Read the model definition and answer for the solid it produces. Units are mm, in the model's axes. A direction names the side the tool comes from. Coordinates: 2 decimals unless noted, no trailing zeros. Write each loop counter-clockwise with the first axis right and the second up, starting at its lowest first coordinate (ties: lowest second). Pieces come first, ordered by that corner, then holes.
(1) Straight lines are drawn through the part: line 1 along Z through (x, y) = (-37, -0.45); line 2 along X through (y, z) = (-1.2, 22.35); line 3 along Y through (x, z) = (66.2, 37.9). For each, find the intervals that lie inside material, in ascending order.
(2) Which of the six approach directions +Z, -Z, +X, -X, +Y, -Y give full straight-line access (tool end or side, diameter ignored) to faces 4 (the flat face through (0, 0, 20.75)), 5 (the flat face through (27, 0, 2)), 6 (the flat face through (67, 0, 24))?
(3) The part is cut by section A-A, the plane y = -0.95. Determine the outline of the cut face in (x, z).
(4) Determine the mould class of faces 1 (the flat face through (-5.1, 0, 23)), 2 (the flat face through (-47, 0, 0)), 3 (the flat face through (-27, 0, 2)) for opening direction Z: pulls with the +Z half, pulls with the -Z half, needs draft (parallel to the pull), parting line crosses it, or undercut.
(5) The part is cut by section B-B, the plane x = 8. Determine the outline of the cut face in (y, z), and give its area (3 significant figures).
(6) Given pin 1 (1.5 mm diameter, centred on x = -1.5, y = 0, fed in from -Z), flat-ended and moving along its own axis, determine where the tip first touches the part or whether it passes through.
```python
from build123d import *

# Parameters (mm, degrees)
SKETCH_1_W          = 134
SKETCH_1_H          = 3
EXTRUDE_1_DEPTH     = 47.9
SKETCH_4_R          = 0.7
SKETCH_4_W          = 10.2
SKETCH_4_H          = 4.7
SKETCH_4_W_2        = 54
SKETCH_4_H_2        = 3
CUT_EXTRUDE_1_DEPTH = 83.416078528
SKETCH_4_3_R        = 1
SKETCH_4_3_R_2      = 0.7
SKETCH_4_3_W        = 10.2
SKETCH_4_3_H        = 4.7
SKETCH_4_3_W_2      = 54
SKETCH_4_3_H_2      = 3
CUT_EXTRUDE_2_DEPTH = 1.5
SKETCH_5_R          = 0.35
CUT_EXTRUDE_3_DEPTH = 1.5
SKETCH_6_R          = 0.35
CUT_EXTRUDE_4_DEPTH = 1.5
SKETCH_7_R          = 0.35
CUT_EXTRUDE_5_DEPTH = 1.5
CUT_EXTRUDE_START   = -132.5
SKETCH_7_3_R        = 0.35
CUT_EXTRUDE_6_DEPTH = 1.5


with BuildPart() as part:
    # 草图1 → 凸台-拉伸1 (new body)
    with BuildSketch(Plane.XY):
        Rectangle(SKETCH_1_W, SKETCH_1_H)
    extrude(amount=EXTRUDE_1_DEPTH)

    # 草图4 → 切除-拉伸1 (cut, through all)
    with BuildSketch(Plane(origin=(0, 1.5, 0), x_dir=(1, 0, 0), z_dir=(0, 1, 0))):
        with Locations(Location((37, -46.4, 0), (0, 0, 270))):
            Circle(SKETCH_4_R)
        with Locations(Location((-37, -46.4, 0), (0, 0, 270))):
            Circle(SKETCH_4_R)
        with Locations((0, -23.1)):
            Rectangle(SKETCH_4_W, SKETCH_4_H)
        with Locations((0, -1.5)):
            Rectangle(SKETCH_4_W_2, SKETCH_4_H_2)
        with Locations(Location((-37, -1.5, 0), (0, 0, 270))):
            Circle(SKETCH_4_R)
        with Locations(Location((37, -1.5, 0), (0, 0, 270))):
            Circle(SKETCH_4_R)
    extrude(amount=-CUT_EXTRUDE_1_DEPTH, mode=Mode.SUBTRACT)

    # 草图4<3> → 切除-拉伸2 (cut)
    # profile 1 of 6: a face of its own
    with BuildSketch(Plane(origin=(0, 1.5, 0), x_dir=(1, 0, 0), z_dir=(0, 1, 0))):
        with Locations(Location((-37, -46.4, 0), (0, 0, 270))):
            Circle(SKETCH_4_3_R)
        with Locations(Location((-37, -46.4, 0), (0, 0, 270))):
            Circle(SKETCH_4_3_R_2, mode=Mode.SUBTRACT)
    # profile 2 of 6: a face of its own
    with BuildSketch(Plane(origin=(0, 1.5, 0), x_dir=(1, 0, 0), z_dir=(0, 1, 0))):
        with Locations(Location((37, -46.4, 0), (0, 0, 270))):
            Circle(SKETCH_4_3_R)
        with Locations(Location((37, -46.4, 0), (0, 0, 270))):
            Circle(SKETCH_4_3_R_2, mode=Mode.SUBTRACT)
    # profile 3 of 6: a face of its own
    with BuildSketch(Plane(origin=(0, 1.5, 0), x_dir=(1, 0, 0), z_dir=(0, 1, 0))):
        with Locations(Location((37, -1.5, 0), (0, 0, 270))):
            Circle(SKETCH_4_3_R)
        with Locations(Location((37, -1.5, 0), (0, 0, 270))):
            Circle(SKETCH_4_3_R_2, mode=Mode.SUBTRACT)
    # profile 4 of 6: a face of its own
    with BuildSketch(Plane(origin=(0, 1.5, 0), x_dir=(1, 0, 0), z_dir=(0, 1, 0))):
        with Locations(Location((-37, -1.5, 0), (0, 0, 270))):
            Circle(SKETCH_4_3_R)
        with Locations(Location((-37, -1.5, 0), (0, 0, 270))):
            Circle(SKETCH_4_3_R_2, mode=Mode.SUBTRACT)
    # profile 5 of 6: a face of its own
    with BuildSketch(Plane(origin=(0, 1.5, 0), x_dir=(1, 0, 0), z_dir=(0, 1, 0))):
        with Locations((0, -23.1)):
            Rectangle(SKETCH_4_3_W, SKETCH_4_3_H)
    # profile 6 of 6: a face of its own
    with BuildSketch(Plane(origin=(0, 1.5, 0), x_dir=(1, 0, 0), z_dir=(0, 1, 0))):
        with Locations((0, -1.5)):
            Rectangle(SKETCH_4_3_W_2, SKETCH_4_3_H_2)
    extrude(amount=-CUT_EXTRUDE_2_DEPTH, mode=Mode.SUBTRACT)

    # 草图5 → 切除-拉伸3 (cut)
    with BuildSketch(Plane.XZ.offset(1.5)):
        with Locations((42.3, 22.35)):
            Circle(SKETCH_5_R)
        with Locations((-42.3, 22.35)):
            Circle(SKETCH_5_R)
    extrude(amount=-CUT_EXTRUDE_3_DEPTH, mode=Mode.SUBTRACT)

    # 草图6 → 切除-拉伸4 (cut)
    with BuildSketch(Plane(origin=(0, 0, 3), x_dir=(-1, 0, 0), z_dir=(0, 0, -1))):
        Circle(SKETCH_6_R)
    extrude(amount=-CUT_EXTRUDE_4_DEPTH, mode=Mode.SUBTRACT)

    # 草图7 → 切除-拉伸5 (cut)
    with BuildSketch(Plane(origin=(67, 0, 0), x_dir=(0, 0, -1), z_dir=(1, 0, 0))):
        with Locations((-10, 0)):
            Circle(SKETCH_7_R)
        with Locations((-37.9, 0)):
            Circle(SKETCH_7_R)
    extrude(amount=-CUT_EXTRUDE_5_DEPTH, mode=Mode.SUBTRACT)

    # 草图7<3> → 切除-拉伸6 (cut)
    with BuildSketch(Plane(origin=(67, 0, 0), x_dir=(0, 0, -1), z_dir=(1, 0, 0)).offset(CUT_EXTRUDE_START)):
        with Locations((-10, 0)):
            Circle(SKETCH_7_3_R)
        with Locations((-37.9, 0)):
            Circle(SKETCH_7_3_R)
    extrude(amount=-CUT_EXTRUDE_6_DEPTH, mode=Mode.SUBTRACT)


solid = part.part
```
Computed:
1. line 1: z = 0 to 0.8, 2.2 to 45.7, 47.1 to 47.9
1. line 2: x = -67 to -42.65, -41.95 to -5.1, 5.1 to 41.95, 42.65 to 67
1. line 3: y = -1.5 to -0.35, 0.35 to 1.5
2. face 4: +Y, -Y
2. face 5: -Z, +Y, -Y
2. face 6: +Z, -Z, +X, +Y, -Y
3. outline: (-67, 0) - (-27, 0) - (-27, 3) - (27, 3) - (27, 0) - (67, 0) - (67, 47.9) - (-67, 47.9) - close; hole circle Ø0.7 at (-42.3, 22.35); hole circle Ø1.4 at (-37, 1.5); hole circle Ø1.4 at (-37, 46.4); hole (-5.1, 20.75) - (5.1, 20.75) - (5.1, 25.45) - (-5.1, 25.45) - close; hole circle Ø1.4 at (37, 1.5); hole circle Ø1.4 at (37, 46.4); hole circle Ø0.7 at (42.3, 22.35)
4. face 1: undercut
4. face 2: pulls with the -Z half
4. face 3: needs draft
5. outline: (-1.5, 3) - (1.5, 3) - (1.5, 47.9) - (-1.5, 47.9) - close
5. area: 135 mm2
6. pin 1: stops at z = 3
